```python
from build123d import *

# Parameters (mm, degrees)
CUT_EXTRUDE1_DEPTH = 3


with BuildPart() as part:
    # Sketch1 → Revolve1 (revolve)
    with BuildSketch(Plane.XY):
        with BuildLine():
            Line((0, 0), (0, 17))
            Line((0, 17), (4, 17))
            Line((4, 17), (4.5, 16.5))
            Line((4.5, 16.5), (4.5, 13))
            Line((4.5, 13), (2.5, 13))
            ThreePointArc((2.5, 13), (2.146446609, 12.853553391), (2, 12.5))
            Line((2, 12.5), (2, 12))
            Line((2, 12), (2.5, 11.5))
            Line((2.5, 11.5), (2.5, 5))
            Line((2.5, 5), (2, 5))
            ThreePointArc((2, 5), (1.505025253, 4.794974747), (1.3, 4.3))
            Line((1.3, 4.3), (1.3, 3.7))
            Line((1.3, 3.7), (2, 3))
            Line((2, 3), (2, 0.7))
            Line((2, 0.7), (1.3, 0))
            Line((1.3, 0), (0, 0))
        make_face()
    revolve(axis=Axis((0, 0, 0), (0, 1, 0)))

    # Sketch2 → Cut-Extrude1 (cut)
    with BuildSketch(Plane(origin=(0, 17, 0), x_dir=(1, 0, 0), z_dir=(0, 1, 0))):
        Polygon((0.721687836, 1.25), (-0.721687836, 1.25), (-1.443375673, 0), (-0.721687836, -1.25), (0.721687836, -1.25), (1.443375673, 0), align=None)
    extrude(amount=-CUT_EXTRUDE1_DEPTH, mode=Mode.SUBTRACT)


solid = part.part
```
Can you work these out from the model? Positions are in its coordinate system, mm. A direction names the side the tool comes from. Coordinates: 2 decimals unless noted, no trailing zeros. Loops run counter-clockwise (first coordinate to the right, second up) from the corner with the lowest first, then second, coordinate; pieces in that order, holes last. Notation, with made-up numbers: (-30, 78.25) - (27, 78.25) arc R29 cw to (27, 107.25) - close; hole circle Ø6 at (-13.5, 60.5). An arc over 180 degrees is marked (long way). Use a Markdown table: item, result.
Item 1: I want a section at B-B on y = 3.25. Please give me the cut outline in (x, z).
Numbers:
| item | result |
|---|---|
| outline | circle Ø3.5 at (0, 0) |
Item 2: If I drill on probe 1 along Y at (x, z) = (-3.5, 1); probe 2 along Z at (x, y) = (0, 2.5); probe 3 along Y at (x, z) = (-2.25, -0.5), over which ranges is the centre line in solid material (lowest first)? Write a range as from..to.
Numbers:
| item | result |
|---|---|
| probe 1 | y = 13..17 |
| probe 2 | z = -2..2 |
| probe 3 | y = 5..11.7, 12.96..17 |
Item 3: We'd pull the mould along Y, two halves only. Please class faces 1 (the face through (-0.434, 12.246, 1.952)), 2 (the face through (0, 0, 0)), 3 (the face through (1.08, 15.52, 0.63)), 4 (the face through (-0.17, 4, -1.29)): released by +Y, released by -Y, zero draft, split by the parting line, or undercut.
Numbers:
| item | result |
|---|---|
| face 1 | undercut |
| face 2 | released by -Y |
| face 3 | zero draft |
| face 4 | undercut |
Item 4: For faces 5 (the face through (-2, 17, 0)), 6 (the face through (0, 14, 0)), 7 (the face through (-0.54, 8.2, 2.44)), which set-ups out of +Z, -Z, +X, -X, +Y, -Y let a thin tool reach every point of the face, with its end or its side?
Numbers:
| item | result |
|---|---|
| face 5 | +Z, -Z, +X, -X, +Y |
| face 6 | +Y |
| face 7 | -Y |
Item 5: Will these pins go through, and if not, where does the flat tip stop? pin 1 (1.5 mm diameter, centred on y = 5, z = 1.5, fed in from -X); pin 2 (1.5 mm diameter, centred on x = 3, y = 6.5, fed in from -Z).
Numbers:
| item | result |
|---|---|
| pin 1 | stops at x = -2.38 |
| pin 2 | stops at z = -1.09 |
